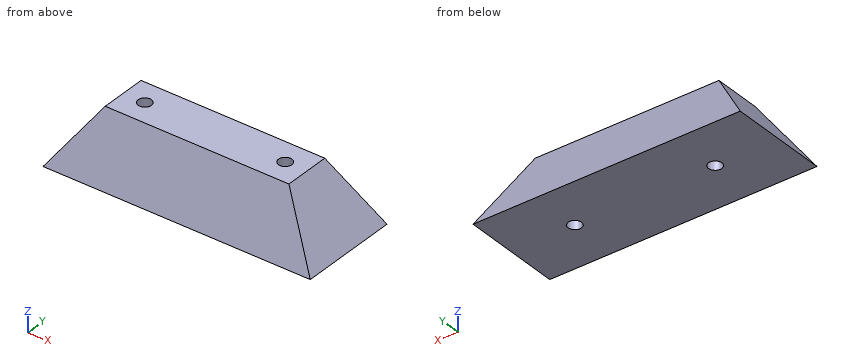
from build123d import *

# Parameters (mm, degrees)
DODANIE_WYCI_GNI_CIE1_DEPTH = 30
WYTNIJ_WYCI_GNI_CIE1_REACH  = 55.141
SZKIC2_R                    = 2
SFAZOWANIE1_SIZE            = 8
SFAZOWANIE1_SIZE_2          = 18
SFAZOWANIE2_SIZE            = 8
SFAZOWANIE2_SIZE_2          = 18


with BuildPart() as part:
    # Szkic1 → Dodanie-wyciągnięcie1 (new body)
    with BuildSketch(Plane(origin=(0, 0, 0), x_dir=(1, 0, 0), z_dir=(0, 1, 0))):
        Polygon((-40, 0), (-27.5, -18), (27.5, -18), (40, 0), align=None)
    extrude(amount=DODANIE_WYCI_GNI_CIE1_DEPTH)

    # Szkic2 → Wytnij-wyciągnięcie1 (cut, up to next)
    with BuildSketch(Plane(origin=(0, 0, 0), x_dir=(-1, 0, 0), z_dir=(0, 0, -1)), mode=Mode.PRIVATE) as wytnij_wyci_gni_cie1_sk1:
        with Locations((-21, 15)):
            Circle(SZKIC2_R)
    wytnij_wyci_gni_cie1_tool1 = extrude(wytnij_wyci_gni_cie1_sk1.sketch, amount=-WYTNIJ_WYCI_GNI_CIE1_REACH, mode=Mode.PRIVATE) & part.part
    # Szkic2 → Wytnij-wyciągnięcie1 (cut, up to next)
    with BuildSketch(Plane(origin=(0, 0, 0), x_dir=(-1, 0, 0), z_dir=(0, 0, -1)), mode=Mode.PRIVATE) as wytnij_wyci_gni_cie1_sk2:
        with Locations((21, 15)):
            Circle(SZKIC2_R)
    wytnij_wyci_gni_cie1_tool2 = extrude(wytnij_wyci_gni_cie1_sk2.sketch, amount=-WYTNIJ_WYCI_GNI_CIE1_REACH, mode=Mode.PRIVATE) & part.part
    add(wytnij_wyci_gni_cie1_tool1.solids().sort_by_distance((21, 15, 0))[0], mode=Mode.SUBTRACT)
    add(wytnij_wyci_gni_cie1_tool2.solids().sort_by_distance((-21, 15, 0))[0], mode=Mode.SUBTRACT)

    # Sfazowanie1
    # the kernel refuses this chamfer: 18, 8 mm, written as the material it takes off along each edge
    with BuildSketch(Plane(origin=(-74.15058918, 0, 18), x_dir=(0, 0.996867139056945, 0.0790942922619672), z_dir=(1, 0, 0))) as sfazowanie1_piece_1:
        Polygon((SFAZOWANIE1_SIZE * 0.996867139057, -SFAZOWANIE1_SIZE * 0.079094292262), (-SFAZOWANIE1_SIZE_2 * 0.079094292262, -SFAZOWANIE1_SIZE_2 * 0.996867139057), (0, 0), align=None)
    extrude(amount=148.301178361, mode=Mode.SUBTRACT)

    # Sfazowanie2
    # the kernel refuses this chamfer: 18, 8 mm, written as the material it takes off along each edge
    with BuildSketch(Plane(origin=(-74.15058918, 30, 18), x_dir=(0, -0.996867139056945, 0.0790942922619672), z_dir=(1, 0, 0))) as sfazowanie2_piece_1:
        Polygon((SFAZOWANIE2_SIZE * 0.996867139057, SFAZOWANIE2_SIZE * 0.079094292262), (-SFAZOWANIE2_SIZE_2 * 0.079094292262, SFAZOWANIE2_SIZE_2 * 0.996867139057), (0, 0), align=None)
    extrude(amount=148.301178361, mode=Mode.SUBTRACT)


solid = part.part
Input: part model. Units: mm. Frame: model coordinates. Give positions to 0.01 mm unless a question says otherwise; leave off trailing zeros. Write each loop counter-clockwise with the first axis right and the second up, starting at its lowest first coordinate (ties: lowest second). Pieces come first, ordered by that corner, then holes. Notation, with made-up numbers: M -22.75,48.25 L 20.25,48.25 A13 cw 20.25,62.25 Z; hole C 50,89.25 d4. An arc over 180 degrees is marked long. Write item = value, one per line. Start each with the question number.
1) Cut plane B-B on x = -21. Return the cut outline in (y, z).
2) Cut plane C-C on z = 7.25. Return the cut outline in (x, y), then the cut area to 3 significant figures.
3) First-contact query: pin 1 Ø1.5 at (x, z) = (-9.5, 6) entering from +Y; pin 2 Ø4 at (y, z) = (20, 2.5) entering from +X; pin 3 Ø6 at (x, z) = (-26, 4.5) entering from -Y; pin 4 Ø3.5 at (x, y) = (-21, 15) entering from +Z. Flat tips, straight axial feed; report the tip coordinate or a pass-through.
4) Material intervals for line 1 along Y through (x, z) = (-21, 5.75); line 2 along Z through (x, y) = (16, 3.5) (3 decimals); line 3 along X through (y, z) = (18, 6.5), sorted ascending. Write a range as [from, to].
5) Cut plane D-D on x = -5.5. Return the cut outline in (y, z), then the cut area to 3 significant figures.
6) Cut plane A-A on y = 15. Return the cut outline in (x, z).
Solved:
q1.outline = M 0,0 L 13,0 L 13,18 L 8,18 Z; M 17,0 L 30,0 L 22,18 L 17,18 Z
q2.outline = M -34.97,3.22 L 34.97,3.22 L 34.97,26.78 L -34.97,26.78 Z; hole C -21,15 d4; hole C 21,15 d4
q2.area = 1,620 mm2
q3.pin_1 = 27.67
q3.pin_2 = 39.65
q3.pin_3 = 0.67
q3.pin_4 = through
q4.line_1 = [2.56, 13], [17, 27.44]
q4.line_2 = [0, 7.875]
q4.line_3 = [-35.49, 35.49]
q5.outline = M 0,0 L 30,0 L 22,18 L 8,18 Z
q5.area = 396 mm2
q6.outline = M -40,0 L -23,0 L -23,18 L -27.5,18 Z; M -19,0 L 19,0 L 19,18 L -19,18 Z; M 23,0 L 40,0 L 27.5,18 L 23,18 Z
